The listing builds one solid part. Answer for the finished solid, in the listing's coordinates (mm). Coordinates: 2 decimals unless noted, no trailing zeros. Order: outer loops, then holes, each group sorted by start corner. A loop starts at its lowest first (then second) coordinate and runs counter-clockwise, first axis right, second up. Notation, with made-up numbers: (7, 14.25) -> (19, 14.25) arc R29 cw to (19, 51.25) -> close; hole circle Ø5 at (-2.75, -18.5). An arc over 180 degrees is marked (long way). One line per question, with ' | ' between items.
Autodesk Fusion 360 part; units mm, degrees
sketch "Sketch1" plane through (0, 0, 0) normal (1, 0, 0) x (0, 1, 0)
  line L0 (-18.3, 27.3) -> (18.3, 27.3)
  line L1 (18.3, 27.3) -> (18.3, -22.3)
  line L2 (13.5, -27.3) -> (-13.5, -27.3)
  line L3 (-18.3, -22.3) -> (-18.3, 27.3)
  line L4 (0, 0) -> (0, 27.3) construction
  line L5 (-13.5, 27.3) -> (-13.5, -22.3) construction
  line L6 (13.5, 27.3) -> (13.5, -22.3) construction
  line L7 (-18.3, 22.5) -> (18.3, 22.5) construction
  line L8 (-18.3, -17.5) -> (18.3, -17.5) construction
  line L9 (-13.5, -22.3) -> (13.5, -22.3) construction
  line L10 (-18.3, 2.5) -> (18.3, 2.5) construction
  line L11 (0, 0) -> (0, -19.9) construction
  circle A0 centre (0, -19.9) radius 1.5
  circle A1 centre (-15.9, 2.5) radius 1.5
  circle A2 centre (15.9, 2.5) radius 1.5
  circle A3 centre (0, 24.9) radius 1.5
  line L12 (-18.3, -22.3) -> (-15.6213, -22.3)
  line L13 (-13.5, -24.4213) -> (-13.5, -27.3)
  line L14 (13.5, -24.4213) -> (13.5, -27.3)
  line L15 (15.6213, -22.3) -> (18.3, -22.3)
  line L16 (-18.3, -27.3) -> (-18.3, -22.3) construction
  line L17 (-13.5, -27.3) -> (-18.3, -27.3) construction
  line L18 (18.3, -27.3) -> (13.5, -27.3) construction
  line L19 (0, 0) -> (18.3, 0)
  line L20 (18.3, -22.3) -> (18.3, -27.3) construction
  line L21 (-13.5, -22.3) -> (-14.5607, -23.3607) construction
  arc A4 (-13.5, -24.4213) -> (-15.6213, -22.3) centre (-14.5607, -23.3607) ccw
  arc A5 (-15.6213, -22.3) -> (-13.5, -24.4213) centre (-14.5607, -23.3607) ccw construction
  line L22 (-13.5, -22.3) -> (-13.5, -24.4213) construction
  line L23 (-15.6213, -22.3) -> (-13.5, -22.3) construction
  line L24 (13.5, -22.3) -> (14.5607, -23.3607) construction
  arc A6 (15.6213, -22.3) -> (13.5, -24.4213) centre (14.5607, -23.3607) ccw
  arc A7 (13.5, -24.4213) -> (15.6213, -22.3) centre (14.5607, -23.3607) ccw construction
  line L25 (13.5, -22.3) -> (15.6213, -22.3) construction
  line L26 (13.5, -22.3) -> (13.5, -24.4213) construction
  line L27 (-15.9, -0.25) -> (-18.3, -0.25)
  line L28 (-15.9, 5.25) -> (-18.3, 5.25)
  arc A8 (-15.9, -0.25) -> (-15.9, 5.25) centre (-15.9, 2.5) ccw
  arc A9 (-15.9, 5.25) -> (-18.3, 3.8426) centre (-15.9, 2.5) ccw construction
  arc A10 (-18.3, 3.8426) -> (-18.3, 1.1574) centre (-15.9, 2.5) ccw construction
  arc A11 (-18.3, 1.1574) -> (-15.9, -0.25) centre (-15.9, 2.5) ccw construction
  line L29 (15.9, 5.25) -> (18.3, 5.25)
  line L30 (15.9, -0.25) -> (18.3, -0.25)
  arc A12 (15.9, -0.25) -> (15.9, 5.25) centre (15.9, 2.5) ccw construction
  arc A13 (14.7544, 0) -> (15.9, -0.25) centre (15.9, 2.5) ccw
  arc A14 (13.5, 1.1574) -> (14.7544, 0) centre (15.9, 2.5) ccw
  arc A15 (13.15, 2.5) -> (13.5, 1.1574) centre (15.9, 2.5) ccw
  arc A16 (13.5, 3.8426) -> (13.15, 2.5) centre (15.9, 2.5) ccw
  arc A17 (15.9, 5.25) -> (13.5, 3.8426) centre (15.9, 2.5) ccw
  point P0 (18.3, 0)
  dimension "d20" = 4.8
  dimension "d21" = 4.8
  dimension "d22" = 4.8
  dimension "d23" = 27
  dimension "d24" = 4.8
  dimension "d25" = 5
  dimension "d26" = 40
  dimension "d27" = 20
  dimension "d28" = 2.4
  dimension "d29" = 3
  dimension "d30" = 3
  dimension "d31" = 3
  dimension "d32" = 3
  dimension "d33" = 2.4
  dimension "d34" = 2.4
  dimension "d35" = 2.4
  dimension "d38" = 2.5
  dimension "d39" = 1.5
  dimension "d40" = 45
  dimension "d41" = 3
  dimension "d42" = 1.5
  dimension "d43" = 45
  dimension "d44" = 3
  dimension "d45" = 5.5
  dimension "d46" = 5.5
extrude "Extrude1" add sketch "Sketch1" along normal blind 4.8
extrude "Extrude2" cut sketch "Sketch1" along normal blind 3 contours L3 L27 L28 A8 | L1 L19 L29 A14 A15 A16 A17 | L1 L19 L30 A13
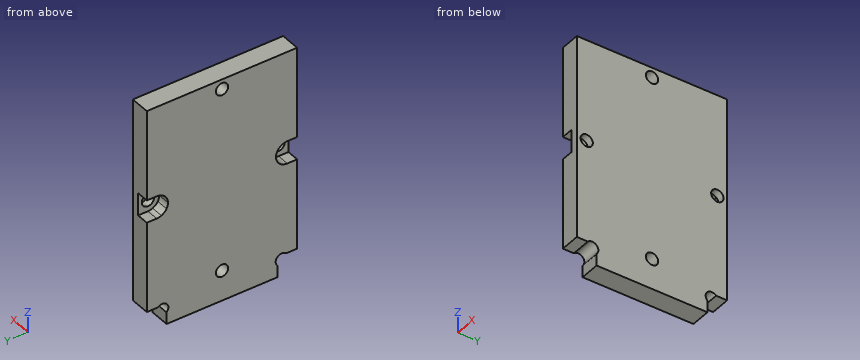
Item 1: Section C-C, the plane x = 1.65 is taken. Give the vertices of the cut face in (y, z), plus the area to 3 significant figures.
Computed values:
outline: (-18.3, -22.3) -> (-15.62, -22.3) arc R1.5 cw to (-13.5, -24.42) -> (-13.5, -27.3) -> (13.5, -27.3) -> (13.5, -24.42) arc R1.5 cw to (15.62, -22.3) -> (18.3, -22.3) -> (18.3, -0.25) -> (15.9, -0.25) arc R2.75 cw to (14.75, 0) arc R2.75 cw to (13.5, 1.16) arc R2.75 cw to (13.15, 2.5) arc R2.75 cw to (13.5, 3.84) arc R2.75 cw to (15.9, 5.25) -> (18.3, 5.25) -> (18.3, 27.3) -> (-18.3, 27.3) -> (-18.3, 5.25) -> (-15.9, 5.25) arc R2.75 cw to (-15.9, -0.25) -> (-18.3, -0.25) -> close; hole circle Ø3 at (0, -19.9); hole circle Ø3 at (0, 24.9) | area: 1,880 mm^2
Item 2: Each of these flat-tipped pins is pushed along its axis until it touches: pin 1 Ø2.5 at (x, y) = (1, -17.5) entering from -Z; pin 2 Ø1.4 at (x, z) = (2, -25.5) entering from +Y; pin 3 Ø1.5 at (y, z) = (15.5, 3.5) entering from -X. Where does it stop, or does it pass through?
Computed values:
pin 1: stops at z = -22.3 | pin 2: stops at y = 13.5 | pin 3: stops at x = 3
Item 3: Section B-B, the plane z = -19.9 is taken. Give the vertices of the cut face in (x, y), plus the area to 3 significant figures.
Computed values:
outline: (0, -18.3) -> (4.8, -18.3) -> (4.8, -1.5) -> (0, -1.5) -> close; (0, 1.5) -> (4.8, 1.5) -> (4.8, 18.3) -> (0, 18.3) -> close | area: 161 mm^2
Item 4: Section A-A, the plane y = 0 is taken. Give the vertices of the cut face in (x, z).
Computed values:
outline: (0, -27.3) -> (4.8, -27.3) -> (4.8, -21.4) -> (0, -21.4) -> close; (0, -18.4) -> (4.8, -18.4) -> (4.8, 23.4) -> (0, 23.4) -> close; (0, 26.4) -> (4.8, 26.4) -> (4.8, 27.3) -> (0, 27.3) -> close
Item 5: Find the intervals of material crossed by L1, parallel to Z at x = 1.75, y = 0; L2, parallel to Z at x = 3.6, y = 15.9; L3, parallel to Y at x = 0.5, z = -20, in increasing order.
Computed values:
L1: z = -27.3 to -21.4, -18.4 to 23.4, 26.4 to 27.3 | L2: z = -22.3 to 1, 4 to 27.3 | L3: y = -18.3 to -1.5, 1.5 to 18.3
